from build123d import *

# Parameters (mm, degrees)
F1_DEPTH      = 1.8
F2_DEPTH      = 4
F2_DEPTH_BACK = 0.1
F3_DEPTH      = 13
F3_DEPTH_BACK = 1.7
F4_W          = 4.4
F4_H          = 4.4
F5_DEPTH      = 10
F6_DEPTH      = 3
F7_DEPTH      = 6


with BuildPart() as f1:
    # F0 (on Top) → F1 (new body)
    with BuildSketch(Plane.XY):
        with BuildLine():
            Line((-13.75, 0), (-16.75, 0))
            ThreePointArc((-16.75, 0), (0, -16.75), (16.75, 0))
            Line((16.75, 0), (13.75, 0))
            Line((13.75, 0), (10.25, 0))
            ThreePointArc((10.25, 0), (0, -10.25), (-10.25, 0))
            Line((-10.25, 0), (-13.75, 0))
        make_face()
        with BuildLine():
            Line((-8.25, 0), (-10.25, 0))
            ThreePointArc((-10.25, 0), (0, -10.25), (10.25, 0))
            Line((10.25, 0), (8.25, 0))
            ThreePointArc((8.25, 0), (0, -8.25), (-8.25, 0))
        make_face()
        with BuildLine():
            Line((8.25, 0), (-8.25, 0))
            ThreePointArc((-8.25, 0), (0, -8.25), (8.25, 0))
        make_face()
    extrude(amount=-F1_DEPTH)

    # F0 (on Top) → F2 (join, two sides)
    with BuildSketch(Plane.XY) as f2_sk:
        with BuildLine():
            ThreePointArc((11.6859958925, 12), (12.7761141335, 10.8320546365), (13.75, 9.5655632349))
            Line((13.75, 9.5655632349), (13.75, 12))
            Line((13.75, 12), (11.6859958925, 12))
        make_face()
        with BuildLine():
            ThreePointArc((-10.0529846314, 2), (-10.2006272472, 1.0048401683), (-10.25, 0))
            Line((-10.25, 0), (-8.25, 0))
            ThreePointArc((-8.25, 0), (-8.1882451935, 1.0075418854), (-8.0039052968, 2))
            Line((-8.0039052968, 2), (-10.0529846314, 2))
        make_face()
        with BuildLine():
            ThreePointArc((-8.0039052968, 2), (-8.1882451935, 1.0075418854), (-8.25, 0))
            Line((-8.25, 0), (8.25, 0))
            ThreePointArc((8.25, 0), (8.1882451935, 1.0075418854), (8.0039052968, 2))
            Line((8.0039052968, 2), (-8.0039052968, 2))
        make_face()
        with BuildLine():
            Line((8.25, 0), (10.25, 0))
            ThreePointArc((10.25, 0), (10.2006272472, 1.0048401683), (10.0529846314, 2))
            Line((10.0529846314, 2), (8.0039052968, 2))
            ThreePointArc((8.0039052968, 2), (8.1882451935, 1.0075418854), (8.25, 0))
        make_face()
        with BuildLine():
            ThreePointArc((-11.6859958925, 12), (-12.7761141335, 10.8320546365), (-13.75, 9.5655632349))
            Line((-13.75, 9.5655632349), (-13.75, 2))
            Line((-13.75, 2), (-10.0529846314, 2))
            ThreePointArc((-10.0529846314, 2), (0, 10.25), (10.0529846314, 2))
            Line((10.0529846314, 2), (13.75, 2))
            Line((13.75, 2), (13.75, 9.5655632349))
            ThreePointArc((13.75, 9.5655632349), (12.7761141335, 10.8320546365), (11.6859958925, 12))
            Line((11.6859958925, 12), (-11.6859958925, 12))
        make_face()
        with BuildLine():
            Line((8.25, 0), (-8.25, 0))
            ThreePointArc((-8.25, 0), (0, -8.25), (8.25, 0))
        make_face()
        with BuildLine():
            Line((-8.25, 0), (-10.25, 0))
            ThreePointArc((-10.25, 0), (0, -10.25), (10.25, 0))
            Line((10.25, 0), (8.25, 0))
            ThreePointArc((8.25, 0), (0, -8.25), (-8.25, 0))
        make_face()
        with BuildLine():
            ThreePointArc((10.0529846314, 2), (0, 10.25), (-10.0529846314, 2))
            Line((-10.0529846314, 2), (-8.0039052968, 2))
            ThreePointArc((-8.0039052968, 2), (0, 8.25), (8.0039052968, 2))
            Line((8.0039052968, 2), (10.0529846314, 2))
        make_face()
        with BuildLine():
            ThreePointArc((8.0039052968, 2), (0, 8.25), (-8.0039052968, 2))
            Line((-8.0039052968, 2), (8.0039052968, 2))
        make_face()
        with BuildLine():
            Line((-13.75, 12), (-13.75, 9.5655632349))
            ThreePointArc((-13.75, 9.5655632349), (-12.7761141335, 10.8320546365), (-11.6859958925, 12))
            Line((-11.6859958925, 12), (-13.75, 12))
        make_face()
    extrude(amount=F2_DEPTH)
    extrude(f2_sk.sketch, amount=-F2_DEPTH_BACK)

    # F0 (on Top) → F3 (join, two sides)
    with BuildSketch(Plane.XY) as f3_sk:
        with BuildLine():
            Line((-8.25, 0), (-10.25, 0))
            ThreePointArc((-10.25, 0), (0, -10.25), (10.25, 0))
            Line((10.25, 0), (8.25, 0))
            ThreePointArc((8.25, 0), (0, -8.25), (-8.25, 0))
        make_face()
    extrude(amount=F3_DEPTH)
    extrude(f3_sk.sketch, amount=-F3_DEPTH_BACK)

    # F4 (on face) → F5 (cut)
    with BuildSketch(Plane.XY.offset(4)):
        with Locations((0, -3.653314048)):
            Rectangle(F4_W, F4_H)
    extrude(amount=-F5_DEPTH, mode=Mode.SUBTRACT)

    # F4 (on face) → F6 (join)
    with BuildSketch(Plane.XY.offset(4)):
        Polygon((-3.55, -0.103314048), (-2.2, -0.103314048), (-2.2, 0.696685952), (-4.35, 0.696685952), (-4.35, -1.453314048), (-3.55, -1.453314048), align=None)
        Polygon((2.2, -0.103314048), (3.55, -0.103314048), (3.55, -1.453314048), (4.35, -1.453314048), (4.35, 0.696685952), (2.2, 0.696685952), align=None)
    extrude(amount=F6_DEPTH)

    # F4 (on face) → F7 (join)
    with BuildSketch(Plane.XY.offset(4)):
        with BuildLine():
            Line((4.0217865093, -7.203314048), (3.55, -7.203314048))
            Line((3.55, -7.203314048), (-3.55, -7.203314048))
            Line((-3.55, -7.203314048), (-4.0217865093, -7.203314048))
            ThreePointArc((-4.0217865093, -7.203314048), (0, -8.25), (4.0217865093, -7.203314048))
        make_face()
    extrude(amount=F7_DEPTH)


solid = f1.part
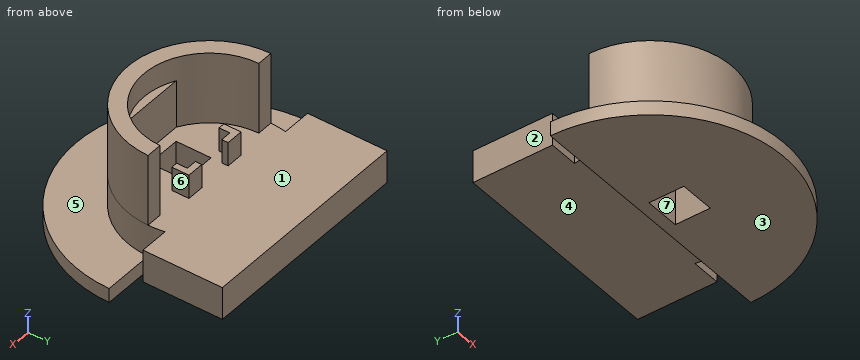
Input: part model. Units: mm. Frame: model coordinates. Face numbers are marked on the shaded views. A direction names the side the tool comes from. Coordinates: 2 decimals unless noted, no trailing zeros. Loops run counter-clockwise (first coordinate to the right, second up) from the corner with the lowest first, then second, coordinate; pieces in that order, holes last. Notation, with made-up numbers: (-35.75, 82) -> (8.25, 82) arc R14 cw to (8.25, 101) -> close; hole circle Ø11 at (-36.5, 85.5). An arc over 180 degrees is marked (long way). Write item = value, one per line. Start each with the question number.
Item 1: Cut plane D-D, the plane z = 9. Return loops of the section in (x, y), plus the area to 3 significant figures.
Item 2: Cut plane A-A, the plane x = 0. Return loops of the section in (y, z), plus the area to 3 significant figures.
Item 3: Cut plane B-B, the plane z = 5.25. Return loops of the section in (x, y), plus the area to 3 significant figures.
Item 4: Mould query, pull axis X, two halves, no side actions, for the marked faces 1, 2 and 3. Classes: pulls with the +X half, pulls with the -X half, needs draft (parallel to the pull), parting line crosses it, or undercut.
Item 5: First-contact query: P1, Ø2.5, axis at x = 3, z = 6, coming from the +Y side; P2, Ø0.9, axis at y = 0.5, z = 6, coming from the +X side; P3, Ø4.5, axis at y = 5, z = 2.5, coming from the +X side. Flat tips, straight axial feed; report the tip coordinate or a pass-through.
Item 6: Material intervals for line 1 (Y direction, x = -2, z = 8.5); line 2 (Z direction, x = -9, y = 4.25); line 3 (X direction, y = -4.5, z = 2), sorted ascending.
Item 7: Cut plane C-C, the plane y = -4.75. Return loops of the section in (x, z), plus the area to 3 significant figures.
Item 8: Reachability of the marked faces 4, 5, 6 and 7 from +Z, -Z, +X, -X, +Y, -Y: full face, straight path, thin tool, end or side. Return the list, or none.
Ans:
q1.outline = (-10.25, 0) arc R10.25 ccw to (10.25, 0) -> (8.25, 0) arc R8.25 cw to (4.02, -7.2) -> (-4.02, -7.2) arc R8.25 cw to (-8.25, 0) -> close
q1.area = 63.8 mm²
q2.outline = (-16.75, -1.8) -> (-5.85, -1.8) -> (-5.85, 4) -> (-7.2, 4) -> (-7.2, 10) -> (-8.25, 10) -> (-8.25, 13) -> (-10.25, 13) -> (-10.25, 0) -> (-16.75, 0) -> close; (-1.45, -1.8) -> (0, -1.8) -> (0, -0.1) -> (12, -0.1) -> (12, 4) -> (-1.45, 4) -> close
q2.area = 119 mm²
q3.outline = (-10.25, 0) arc R10.25 ccw to (10.25, 0) -> (8.25, 0) arc R8.25 cw to (4.02, -7.2) -> (-4.02, -7.2) arc R8.25 cw to (-8.25, 0) -> close; (-4.35, -1.45) -> (-3.55, -1.45) -> (-3.55, -0.1) -> (-2.2, -0.1) -> (-2.2, 0.7) -> (-4.35, 0.7) -> close; (2.2, -0.1) -> (3.55, -0.1) -> (3.55, -1.45) -> (4.35, -1.45) -> (4.35, 0.7) -> (2.2, 0.7) -> close
q3.area = 69.4 mm²
q4.face_1 = undercut
q4.face_2 = pulls with the -X half
q4.face_3 = needs draft
q5.P1 = 0.7
q5.P2 = 4.35
q5.P3 = 13.75
q6.line_1 = -10.05 to -7.2
q6.line_2 = -0.1 to 4
q6.line_3 = -9.21 to -2.2, 2.2 to 9.21
q7.outline = (-16.06, -1.8) -> (-2.2, -1.8) -> (-2.2, 4) -> (-6.75, 4) -> (-6.75, 13) -> (-9.08, 13) -> (-9.08, 0) -> (-16.06, 0) -> close; (2.2, -1.8) -> (16.06, -1.8) -> (16.06, 0) -> (9.08, 0) -> (9.08, 13) -> (6.75, 13) -> (6.75, 4) -> (2.2, 4) -> close
q7.area = 147 mm²
q8.face_4 = -Z, +X, -X, +Y
q8.face_5 = +Z, -Y
q8.face_6 = +Z, +Y
q8.face_7 = +Z, -Z
